from build123d import *

# Parameters (mm, degrees)
F2_W     = 8
F2_H     = 8
F3_DEPTH = 5
F2_W_2   = 20
F2_H_2   = 10
F2_H_3   = 2
F2_W_3   = 10
F2_H_4   = 20
F2_W_4   = 2
F2_W_5   = 95
F2_H_5   = 87.5
F4_DEPTH = 1


with BuildPart() as f3:
    # F2 (on Top) → F3 (new body)
    with BuildSketch(Plane.XY):
        Polygon((-105, 117.5), (-125, 117.5), (-125, 97.5), (-115, 97.5), (-115, 107.5), (-105, 107.5), align=None)
        Polygon((-105, 105.5), (-105, 107.5), (-115, 107.5), (-115, 97.5), (-113, 97.5), (-113, 105.5), align=None)
        with Locations((-109, 101.5)):
            Rectangle(F2_W, F2_H)
    extrude(amount=F3_DEPTH)



with BuildPart() as f3b:
    # F2 (on Top) → F3, piece 2 (new body)
    with BuildSketch(Plane.XY):
        with Locations((0, 112.5)):
            Rectangle(F2_W_2, F2_H_2)
        with Locations((0, 106.5)):
            Rectangle(F2_W_2, F2_H_3)
        Polygon((10, 105.5), (-10, 105.5), (-10, 97.5), (0, 97.5), (2, 97.5), (10, 97.5), align=None)
    extrude(amount=F3_DEPTH)


with BuildPart() as f3c:
    # F2 (on Top) → F3, piece 3 (new body)
    with BuildSketch(Plane.XY):
        Polygon((105, 117.5), (105, 107.5), (115, 107.5), (115, 97.5), (125, 97.5), (125, 117.5), align=None)
        Polygon((115, 107.5), (105, 107.5), (105, 105.5), (113, 105.5), (113, 97.5), (115, 97.5), align=None)
        with Locations((109, 101.5)):
            Rectangle(F2_W, F2_H)
    extrude(amount=F3_DEPTH)


with BuildPart() as f3d:
    # F2 (on Top) → F3, piece 4 (new body)
    with BuildSketch(Plane.XY):
        with Locations((-120, 0)):
            Rectangle(F2_W_3, F2_H_4)
        with Locations((-114, 0)):
            Rectangle(F2_W_4, F2_H_4)
        Polygon((-105, 10), (-113, 10), (-113, -10), (-105, -10), (-105, -2), (-105, 0), align=None)
    extrude(amount=F3_DEPTH)


with BuildPart() as f3e:
    # F2 (on Top) → F3, piece 5 (new body)
    with BuildSketch(Plane.XY):
        with Locations((-5, -6)):
            Rectangle(F2_W_3, F2_H)
        with Locations((-5, -1)):
            Rectangle(F2_W_3, F2_H_3)
        with Locations((-5, 5)):
            Rectangle(F2_W_3, F2_H_2)
        with Locations((6, 5)):
            Rectangle(F2_W, F2_H_2)
        with Locations((1, 5)):
            Rectangle(F2_W_4, F2_H_2)
        with Locations((1, -6)):
            Rectangle(F2_W_4, F2_H)
        with Locations((6, -6)):
            Rectangle(F2_W, F2_H)
        with Locations((6, -1)):
            Rectangle(F2_W, F2_H_3)
    extrude(amount=F3_DEPTH)


with BuildPart() as f3f:
    # F2 (on Top) → F3, piece 6 (new body)
    with BuildSketch(Plane.XY):
        Polygon((113, -10), (113, 10), (105, 10), (105, 0), (105, -2), (105, -10), align=None)
        with Locations((114, 0)):
            Rectangle(F2_W_4, F2_H_4)
        with Locations((120, 0)):
            Rectangle(F2_W_3, F2_H_4)
    extrude(amount=F3_DEPTH)


with BuildPart() as f3g:
    # F2 (on Top) → F3, piece 7 (new body)
    with BuildSketch(Plane.XY):
        Polygon((-115, -107.5), (-115, -97.5), (-125, -97.5), (-125, -117.5), (-105, -117.5), (-105, -107.5), align=None)
        Polygon((-113, -97.5), (-115, -97.5), (-115, -107.5), (-105, -107.5), (-105, -105.5), (-113, -105.5), align=None)
        with Locations((-109, -101.5)):
            Rectangle(F2_W, F2_H)
    extrude(amount=F3_DEPTH)


with BuildPart() as f3h:
    # F2 (on Top) → F3, piece 8 (new body)
    with BuildSketch(Plane.XY):
        with Locations((0, -112.5)):
            Rectangle(F2_W_2, F2_H_2)
        with Locations((0, -106.5)):
            Rectangle(F2_W_2, F2_H_3)
        Polygon((-10, -97.5), (-10, -105.5), (10, -105.5), (10, -97.5), (2, -97.5), (0, -97.5), align=None)
    extrude(amount=F3_DEPTH)


with BuildPart() as f3i:
    # F2 (on Top) → F3, piece 9 (new body)
    with BuildSketch(Plane.XY):
        Polygon((125, -97.5), (115, -97.5), (115, -107.5), (105, -107.5), (105, -117.5), (125, -117.5), align=None)
        Polygon((115, -107.5), (115, -97.5), (113, -97.5), (113, -105.5), (105, -105.5), (105, -107.5), align=None)
        with Locations((109, -101.5)):
            Rectangle(F2_W, F2_H)
    extrude(amount=F3_DEPTH)


with BuildPart() as f3_1:
    add(f3.part)

    add(f3b.part)  # F4 merges F3b

    add(f3c.part)  # F4 merges F3c

    add(f3d.part)  # F4 merges F3d

    add(f3e.part)  # F4 merges F3e

    add(f3f.part)  # F4 merges F3f

    add(f3g.part)  # F4 merges F3g

    add(f3h.part)  # F4 merges F3h

    add(f3i.part)  # F4 merges F3i
    # F2 (on Top) → F4 (join)
    with BuildSketch(Plane.XY):
        with Locations((-57.5, 106.5)):
            Rectangle(F2_W_5, F2_H_3)
        with Locations((57.5, 106.5)):
            Rectangle(F2_W_5, F2_H_3)
        with Locations((114, 53.75)):
            Rectangle(F2_W_4, F2_H_5)
        with Locations((114, -53.75)):
            Rectangle(F2_W_4, F2_H_5)
        with Locations((57.5, -106.5)):
            Rectangle(F2_W_5, F2_H_3)
        with Locations((-57.5, -106.5)):
            Rectangle(F2_W_5, F2_H_3)
        with Locations((-114, -53.75)):
            Rectangle(F2_W_4, F2_H_5)
        with Locations((-114, 53.75)):
            Rectangle(F2_W_4, F2_H_5)
        with Locations((1, 53.75)):
            Rectangle(F2_W_4, F2_H_5)
        with Locations((1, -53.75)):
            Rectangle(F2_W_4, F2_H_5)
        with Locations((-57.5, -1)):
            Rectangle(F2_W_5, F2_H_3)
        with Locations((57.5, -1)):
            Rectangle(F2_W_5, F2_H_3)
    extrude(amount=F4_DEPTH)


solid = f3_1.part
The listing builds one solid part. Answer for the finished solid, in the listing's coordinates (mm). Give positions to 0.01 mm unless a question says otherwise; leave off trailing zeros. Write each loop counter-clockwise with the first axis right and the second up, starting at its lowest first coordinate (ties: lowest second). Pieces come first, ordered by that corner, then holes.
Item 1: Find the intervals of material crossed by line 1 along X through (y, z) = (-83, 0.75); line 2 along Y through (x, z) = (-111.5, 0.6); line 3 along Y through (x, z) = (-71.5, 0.75), in increasing order.
Item 2: Section B-B, the plane y = -33.5 is taken. Write down the section's boundary in (x, z).
Item 3: Section C-C, the plane z = 3.9 is taken. Count the separate pieces of the cut face and the enclosed holes in it, plus the area to 3 significant figures.
Item 4: Section A-A, the plane x = -20 is taken. Write down the section's boundary in (y, z).
Item 5: Flat-ended cylindrical pins translate along their axes: P1, Ø0.8, axis at x = 46.5, z = 0.5, coming from the +Y side; P2, Ø0.8, axis at y = -70.5, z = 0.5, coming from the +X side; P3, Ø1.6, axis at x = 69.5, y = 106.5, coming from the +Z side. Find the tip coordinate at first contact, or state that the pin passes through.
Completed:
1. line 1: x = -115 to -113, 0 to 2, 113 to 115
1. line 2: y = -117.5 to -97.5, -10 to 10, 97.5 to 117.5
1. line 3: y = -107.5 to -105.5, -2 to 0, 105.5 to 107.5
2. outline: (-115, 0) - (-113, 0) - (-113, 1) - (-115, 1) - close; (0, 0) - (2, 0) - (2, 1) - (0, 1) - close; (113, 0) - (115, 0) - (115, 1) - (113, 1) - close
3. separate pieces: 9
3. enclosed holes: 1
3. area: 3,600 mm2
4. outline: (-107.5, 0) - (-105.5, 0) - (-105.5, 1) - (-107.5, 1) - close; (-2, 0) - (0, 0) - (0, 1) - (-2, 1) - close; (105.5, 0) - (107.5, 0) - (107.5, 1) - (105.5, 1) - close
5. P1: stops at y = 107.5
5. P2: stops at x = 115
5. P3: stops at z = 1
